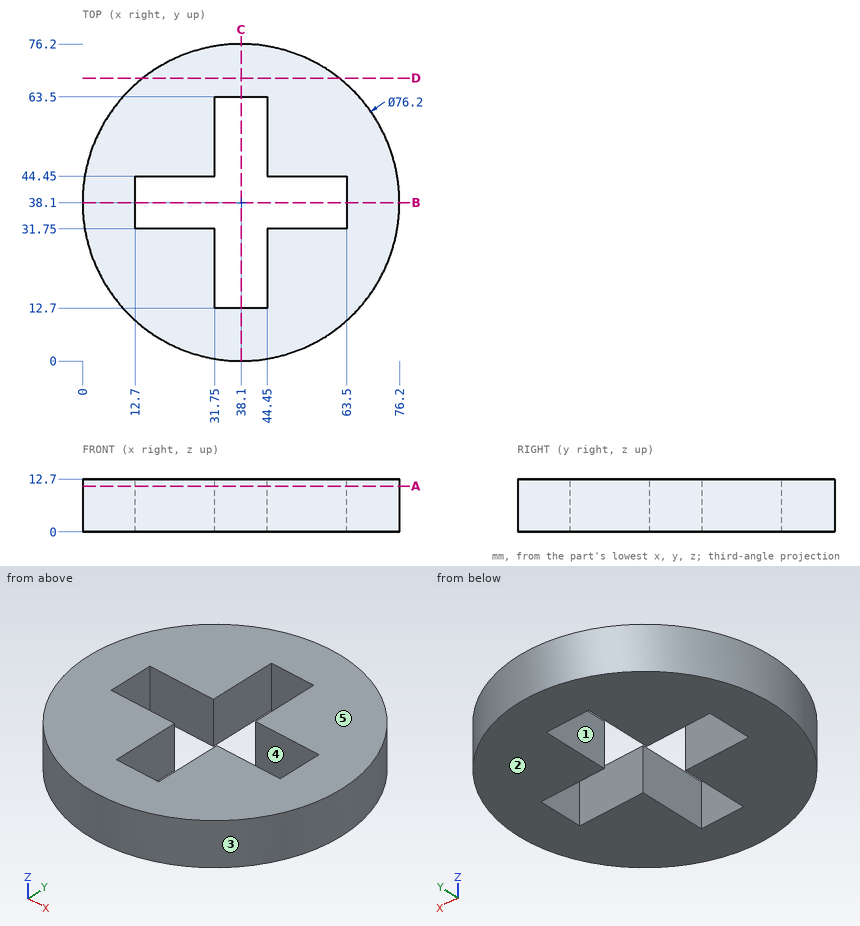
Check sheet for the drawn part. Datum: minimum x, y, z corner. Units: mm. A direction names the side the tool comes from. Give positions to 0.01 mm unless a question says otherwise; leave off trailing zeros. Write each loop counter-clockwise with the first axis right and the second up, starting at its lowest first coordinate (ties: lowest second). Pieces come first, ordered by that corner, then holes.
(1) Mould release check, pull along Y, two halves, no side actions. Record for the marked faces 1, 2 and 3: +Y half, -Y half, draft (parallel to the pull), parting line (faces both ways), or undercut.
(2) Cross-section at D-D (y = 68). Enter the section's corners in (x, z).
(3) Material ranges on line 1 (X direction, y = 37.5, z = 4.75); line 2 (Y direction, x = 50.5, z = 12.25), recorded low to high.
(4) Gauge pin test, flat ends, axial feed: pin 1 (2 mm diameter, centred on y = 16.5, z = 9, fed in from -X); pin 2 (1 mm diameter, centred on y = 7.5, z = 7, fed in from +X); pin 3 (4 mm diameter, centred on x = 56, z = 8.5, fed in from -Y). Record the tip position at first contact, or that the pin passes through.
(5) Cross-section at B-B (y = 38.1). Enter the section's corners in (x, z), plus the area to 3 significant figures.
(6) Access from +Z, -Z, +X, -X, +Y, -Y to the whole of each face (thin tool, end or side, straight path). Record for the marked faces 4 and 5.
(7) Cross-section at A-A (z = 11). Enter the section's corners in (x, y), plus the area to 3 significant figures.
Worked out:
1. face 1: undercut
1. face 2: draft
1. face 3: parting line
2. outline: (14.49, 0) - (61.71, 0) - (61.71, 12.7) - (14.49, 12.7) - close
3. line 1: x = 0 to 12.7, 63.5 to 76.2
3. line 2: y = 2.07 to 31.75, 44.45 to 74.13
4. pin 1: stops at x = 6.05
4. pin 2: stops at x = 61.46
4. pin 3: stops at y = 3.48
5. outline: (0, 0) - (12.7, 0) - (12.7, 12.7) - (0, 12.7) - close; (63.5, 0) - (76.2, 0) - (76.2, 12.7) - (63.5, 12.7) - close
5. area: 323 mm2
6. face 4: +Z, -Z
6. face 5: +Z, +X, -X, +Y, -Y
7. outline: circle Ø76.2 at (38.1, 38.1); hole (12.7, 31.75) - (31.75, 31.75) - (31.75, 12.7) - (44.45, 12.7) - (44.45, 31.75) - (63.5, 31.75) - (63.5, 44.45) - (44.45, 44.45) - (44.45, 63.5) - (31.75, 63.5) - (31.75, 44.45) - (12.7, 44.45) - close
7. area: 3,430 mm2
